Verification items for the finished model (mm, model axes). Face numbers are marked on the shaded views. A direction names the side the tool comes from. Coordinates: 2 decimals unless noted, no trailing zeros. Write each loop counter-clockwise with the first axis right and the second up, starting at its lowest first coordinate (ties: lowest second). Pieces come first, ordered by that corner, then holes. Notation, with made-up numbers: (8, 28.25) -> (21, 28.25) arc R10 cw to (21, 38.25) -> close; hole circle Ø1 at (-39.75, -23.5). An arc over 180 degrees is marked (long way). Answer in a Markdown table with one row per item.
```python
from build123d import *

# Parameters (mm, degrees)
F0_W     = 60.96
F0_H     = 104.14
F0_R     = 17.78
F0_W_2   = 44.47266
F0_H_2   = 38.1
F1_DEPTH = 10.414
F0_R_2   = 7.62
F2_DEPTH = 9.906
F3_DEPTH = 9.398
F4_W     = 16.026364
F4_H     = 2.950886
F5_DEPTH = 5.08
F4_R     = 2.481019
F6_DEPTH = 12.7
F7_R     = 5.08
F8_W     = 28.981276
F8_H     = 3.993245
F9_DEPTH = 12.7


with BuildPart() as f1:
    # F0 (on Top) → F1 (new body)
    with BuildSketch(Plane.XY):
        with Locations((-2.628636, -5.107779)):
            Rectangle(F0_W, F0_H)
        with Locations((-2.628636, -26.697779)):
            Circle(F0_R, mode=Mode.SUBTRACT)
        with Locations((-2.133989, 21.562221)):
            Rectangle(F0_W_2, F0_H_2, mode=Mode.SUBTRACT)
    extrude(amount=F1_DEPTH)

    # F0 (on Top) → F2 (join)
    with BuildSketch(Plane.XY):
        with Locations((-2.133989, 21.562221)):
            Rectangle(F0_W_2, F0_H_2)
        with Locations((-2.628636, -26.697779)):
            Circle(F0_R)
        with Locations((-2.628636, -26.697779)):
            Circle(F0_R_2, mode=Mode.SUBTRACT)
    extrude(amount=F2_DEPTH)

    # F0 (on Top) → F3 (join)
    with BuildSketch(Plane.XY):
        with Locations((-2.628636, -26.697779)):
            Circle(F0_R_2)
    extrude(amount=F3_DEPTH)

    # F4 (on face) → F5 (cut)
    with BuildSketch(Plane(origin=(0, 46.962221, 0), x_dir=(-1, 0, 0), z_dir=(0, 1, 0))):
        with Locations((-14.351097, 5.28416)):
            Rectangle(F4_W, F4_H)
    extrude(amount=-F5_DEPTH, mode=Mode.SUBTRACT)

    # F4 (on face) → F6 (cut)
    with BuildSketch(Plane(origin=(0, 46.962221, 0), x_dir=(-1, 0, 0), z_dir=(0, 1, 0))):
        with Locations((25.215648, 5.702663)):
            Circle(F4_R)
    extrude(amount=-F6_DEPTH, mode=Mode.SUBTRACT)

    # F7
    f7_edges = [f1.edges().sort_by_distance(p)[0] for p in [
        (-33.108636, 46.962221, 5.207),
        (27.851364, 46.962221, 5.207),
        (27.851364, -57.177779, 5.207),
        (-33.108636, -57.177779, 5.207),
    ]]
    fillet(f7_edges, radius=F7_R)

    # F8 (on face) → F9 (cut)
    with BuildSketch(Plane.XZ.offset(57.177779)):
        with Locations((-1.75176, 4.668219)):
            Rectangle(F8_W, F8_H)
    extrude(amount=-F9_DEPTH, mode=Mode.SUBTRACT)


solid = f1.part
```
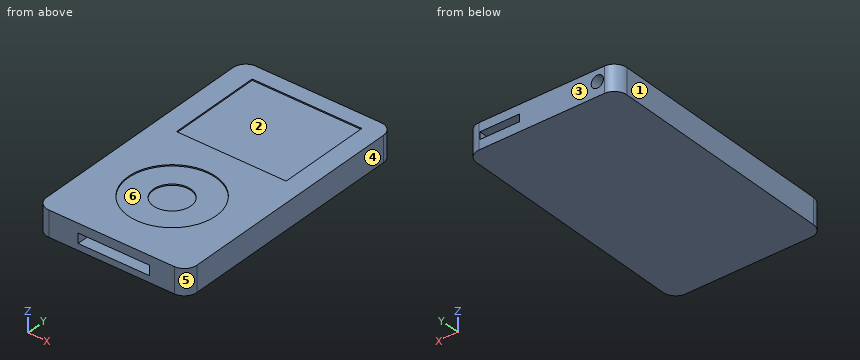
1. Sectioned sample at B-B, the plane x = -3. Record the cut outline in (y, z).
Findings below:
| item | result |
|---|---|
| outline | (-57.18, 0) -> (46.96, 0) -> (46.96, 10.41) -> (40.61, 10.41) -> (40.61, 9.91) -> (2.51, 9.91) -> (2.51, 10.41) -> (-8.92, 10.41) -> (-8.92, 9.91) -> (-19.09, 9.91) -> (-19.09, 9.4) -> (-34.31, 9.4) -> (-34.31, 9.91) -> (-44.47, 9.91) -> (-44.47, 10.41) -> (-57.18, 10.41) -> (-57.18, 6.66) -> (-44.48, 6.66) -> (-44.48, 2.67) -> (-57.18, 2.67) -> close |
2. Sectioned sample at D-D, the plane x = -19. Record the cut outline in (y, z), and give its area (3 significant figures).
Findings below:
| item | result |
|---|---|
| outline | (-57.18, 0) -> (46.96, 0) -> (46.96, 10.41) -> (40.61, 10.41) -> (40.61, 9.91) -> (2.51, 9.91) -> (2.51, 10.41) -> (-19.76, 10.41) -> (-19.76, 9.91) -> (-33.63, 9.91) -> (-33.63, 10.41) -> (-57.18, 10.41) -> close |
| area | 1,060 mm² |
3. Sectioned sample at A-A, the plane y = 32. Record the cut outline in (x, z).
Findings below:
| item | result |
|---|---|
| outline | (-33.11, 0) -> (27.85, 0) -> (27.85, 10.41) -> (20.1, 10.41) -> (20.1, 9.91) -> (-24.37, 9.91) -> (-24.37, 10.41) -> (-33.11, 10.41) -> close |
4. Material ranges on probe 1 along X at (y, z) = (-46, 3.75); probe 2 along Z at (x, y) = (-4, -49); probe 3 along Z at (x, y) = (-7, 15.5), recorded low to high. Write a range as from..to.
Findings below:
| item | result |
|---|---|
| probe 1 | x = -33.11..-16.24, 12.74..27.85 |
| probe 2 | z = 0..2.67, 6.66..10.41 |
| probe 3 | z = 0..9.91 |
5. Access from +Z, -Z, +X, -X, +Y, -Y to the whole of each face (thin tool, end or side, straight path). Record for the marked faces 5 and 6.
Findings below:
| item | result |
|---|---|
| face 5 | +Z, -Z, +X, -Y |
| face 6 | +Z |
6. Go/stop test with flat-tipped pins: pin 1 (12 mm diameter, centred on x = 14.5, y = 14.5, fed in from +Z); pin 2 (19 mm diameter, centred on x = 1, y = 21.5, fed in from +Z); pin 3 (0.9 mm diameter, centred on x = 13.5, z = 5, fed in from +Y); pin 4 (1.5 mm diameter, centred on x = -26, z = 5.5, fed in from +Y). Record where each tip stops, or that it passes through.
Findings below:
| item | result |
|---|---|
| pin 1 | stops at z = 10.41 |
| pin 2 | stops at z = 9.91 |
| pin 3 | stops at y = 41.88 |
| pin 4 | stops at y = 34.26 |
7. Sectioned sample at C-C, the plane y = -38. Record the cut outline in (x, z).
Findings below:
| item | result |
|---|---|
| outline | (-33.11, 0) -> (27.85, 0) -> (27.85, 10.41) -> (11.1, 10.41) -> (11.1, 9.91) -> (-16.35, 9.91) -> (-16.35, 10.41) -> (-33.11, 10.41) -> close |
8. Release check for a two-part mould opening along X. For the marked faces 1, 2, 3 and 4 record: released by +X, released by -X, zero draft, split by the parting line, or undercut.
Findings below:
| item | result |
|---|---|
| face 1 | released by -X |
| face 2 | undercut |
| face 3 | zero draft |
| face 4 | released by +X |
